CAD build for the part. Positions are in the model's coordinates, mm. A direction names the side the tool comes from. Round coordinates to 2 decimals unless told otherwise and drop trailing zeros. Loops run counter-clockwise (first coordinate to the right, second up) from the corner with the lowest first, then second, coordinate; pieces in that order, holes last. Notation, with made-up numbers: M -29,31 L 22,31 A13 ccw 22,41 Z; hole C 13,37.25 d8. An arc over 180 degrees is marked long. One line per item, written item: value. Start each with the question number.
from build123d import *

# Parameters (mm, degrees)
SCHIZZO1_R                   = 12.1
ESTRUSIONE_ESTRUSIONE1_DEPTH = 1
ESTRUSIONE_ESTRUSIONE2_START = -1.8
SCHIZZO2_R                   = 12.1
SCHIZZO2_R_2                 = 9
ESTRUSIONE_ESTRUSIONE2_DEPTH = 1.8
SCHIZZO3_R                   = 1.925
ESTRUSIONE_ESTRUSIONE3_DEPTH = 11
SCHIZZO4_R                   = 1.7
TAGLIO_ESTRUSIONE1_DEPTH     = 2
TAGLIO_ESTRUSIONE2_START     = -7.2
SCHIZZO5_R                   = 1.925
TAGLIO_ESTRUSIONE2_DEPTH     = 7.2
SCHIZZO6_R                   = 1.425
ESTRUSIONE_ESTRUSIONE4_DEPTH = 3.4
SCHIZZO7_R                   = 1.925
ESTRUSIONE_ESTRUSIONE5_DEPTH = 3.8


with BuildPart() as part:
    # Schizzo1 → Estrusione-Estrusione1 (new body)
    with BuildSketch(Plane.XY):
        with BuildLine():
            Line((-6.171311325, 16.1), (6.171311325, 16.1))
            ThreePointArc((6.171311325, 16.1), (13.651991863, 12.73622021), (16.1, 4.907883736))
            Line((16.1, 4.907883736), (16.1, -13.463208293))
            ThreePointArc((16.1, -13.463208293), (14.572915114, -17.149917336), (10.886206072, -18.677002221))
            Line((10.886206072, -18.677002221), (-10.957517396, -18.677002221))
            ThreePointArc((-10.957517396, -18.677002221), (-14.644226439, -17.149917336), (-16.171311325, -13.463208293))
            Line((-16.171311325, -13.463208293), (-16.171311325, 6.1))
            ThreePointArc((-16.171311325, 6.1), (-13.242379137, 13.171067812), (-6.171311325, 16.1))
        make_face()
        Circle(SCHIZZO1_R, mode=Mode.SUBTRACT)
    extrude(amount=ESTRUSIONE_ESTRUSIONE1_DEPTH)

    # Schizzo2 → Estrusione-Estrusione2 (add)
    with BuildSketch(Plane.XY.offset(1).offset(ESTRUSIONE_ESTRUSIONE2_START)):
        Circle(SCHIZZO2_R)
        Circle(SCHIZZO2_R_2, mode=Mode.SUBTRACT)
    extrude(amount=ESTRUSIONE_ESTRUSIONE2_DEPTH)

    # Schizzo3 → Estrusione-Estrusione3 (add)
    with BuildSketch(Plane(origin=(0, 0, 0), x_dir=(-1, 0, 0), z_dir=(0, 0, -1))):
        with Locations(Location((-10.944459062, 10.817992606, 0), (0, 0, 180))):
            Circle(SCHIZZO3_R)
        with Locations(Location((10.910719744, 10.851964601, 0), (0, 0, 180))):
            Circle(SCHIZZO3_R)
        with Locations(Location((0, -15.38859776, 0), (0, 0, 180))):
            Circle(SCHIZZO3_R)
    extrude(amount=ESTRUSIONE_ESTRUSIONE3_DEPTH)

    # Schizzo4 → Taglio-Estrusione1 (cut)
    with BuildSketch(Plane(origin=(0, 12.776964601, 0), x_dir=(1, 0, 0), z_dir=(0, 1, 0))):
        with BuildLine():
            ThreePointArc((-9.045346347, 5.425199137), (-9.603228747, 6.684392286), (-10.910719744, 7.117136381))
            Line((-10.910719744, 7.117136381), (-10.910719744, 3.733261892))
            ThreePointArc((-10.910719744, 3.733261892), (-9.603228747, 4.166005987), (-9.045346347, 5.425199137))
        make_face()
        with BuildLine():
            Line((-10.910719744, 3.733261892), (-10.910719744, 7.117136381))
            ThreePointArc((-10.910719744, 7.117136381), (-12.445346347, 5.425199137), (-10.910719744, 3.733261892))
        make_face()
        with Locations(Location((10.944459062, 5.5, 0), (0, 0, 270))):
            Circle(SCHIZZO4_R)
    extrude(amount=-TAGLIO_ESTRUSIONE1_DEPTH, mode=Mode.SUBTRACT)

    # Schizzo5 → Taglio-Estrusione2 (cut)
    with BuildSketch(Plane(origin=(0, 0, -11), x_dir=(-1, 0, 0), z_dir=(0, 0, -1)).offset(TAGLIO_ESTRUSIONE2_START)):
        with Locations(Location((0, -15.38859776, 0), (0, 0, 180))):
            Circle(SCHIZZO5_R)
    extrude(amount=TAGLIO_ESTRUSIONE2_DEPTH, mode=Mode.SUBTRACT)

    # Schizzo6 → Estrusione-Estrusione4 (add)
    with BuildSketch(Plane(origin=(0, 0, -3.8), x_dir=(-1, 0, 0), z_dir=(0, 0, -1))):
        with Locations((0, -15.38859776)):
            Circle(SCHIZZO6_R)
    extrude(amount=ESTRUSIONE_ESTRUSIONE4_DEPTH)

    # Schizzo7 → Estrusione-Estrusione5 (add)
    with BuildSketch(Plane(origin=(0, 0, -7.2), x_dir=(-1, 0, 0), z_dir=(0, 0, -1))):
        with Locations(Location((0, -15.38859776, 0), (0, 0, 180))):
            Circle(SCHIZZO7_R)
    extrude(amount=ESTRUSIONE_ESTRUSIONE5_DEPTH)


solid = part.part
(1) Flat gauge pins, fed straight in: P1, Ø6, axis at x = 6.5, y = -1.5, coming from the -Z side; P2, Ø2, axis at x = 10.94, z = -5.5, coming from the +Y side; P3, Ø3, axis at y = -5.5, z = -2, coming from the +X side; P4, Ø6, axis at y = -7, z = -6.5, coming from the -X side. Where does each tip first touch, or does it go through?
(2) Which spindle directions (+Z, -Z, +X, -X, +Y, -Y) get a long thin tool onto all of the face, cutting with end or side? Do faces 1 (the flat face through (0, -17, -3.8)), 2 (the flat face through (0.1, -18.677, 0.5)), 3 (the cylindrical face through (-11.161, 8.943, -5.423)). Say none if no direction does.
(3) Slice it at B-B, the plane y = 0. List the corners of the cut face in (x, z), and give its area (3 significant figures).
(4) Slice it at A-A, the plane x = 0. List the corners of the cut face in (y, z), and give its area (3 significant figures).
(5) Mould opens along X. For faces 4 (the flat face through (16.1, -4.1, 0.5)), 5 (the cylindrical face through (10.69, 8.91, -5.42)), 6 (the flat face through (0, -17, -7.2)), 7 (the cylindrical face through (-1.172, 8.923, 0.087)) say: pulls with the +X half, pulls with the -X half, needs draft (parallel to the pull), parting line crosses it, or undercut.
(6) Probe L1, parallel to Y at x = 0, z = -0.05; L2, parallel to Z at x = -8.5, y = -7; L3, parallel to Y at x = 0, z = 0.1. List the from-to ranges inside material, lowest first.
(7) Slice it at C-C, the plane z = -4.5. List the corners of the cut face in (x, y) (3 decimals), and give its area (3 significant figures).
(8) Slice it at D-D, the plane x = -7.5. List the corners of the cut face in (y, z), and give its area (3 significant figures).
Check result:
1. P1: stops at z = -0.8
1. P2: stops at y = 10.78
1. P3: stops at x = 11.19
1. P4: passes through
2. face 1: none
2. face 2: +Z, -Z, +X, -X, -Y
2. face 3: -Z
3. outline: M -16.17,0 L -12.1,0 L -12.1,-0.8 L -9,-0.8 L -9,1 L -16.17,1 Z; M 9,-0.8 L 12.1,-0.8 L 12.1,0 L 16.1,0 L 16.1,1 L 9,1 Z
3. area: 19.2 mm^2
4. outline: M -18.68,0 L -17.31,0 L -17.31,-3.8 L -16.81,-3.8 L -16.81,-7.2 L -17.31,-7.2 L -17.31,-11 L -13.46,-11 L -13.46,-7.2 L -13.96,-7.2 L -13.96,-3.8 L -13.46,-3.8 L -13.46,0 L -12.1,0 L -12.1,-0.8 L -9,-0.8 L -9,1 L -18.68,1 Z; M 9,-0.8 L 12.1,-0.8 L 12.1,0 L 16.1,0 L 16.1,1 L 9,1 Z
4. area: 60.7 mm^2
5. face 4: pulls with the +X half
5. face 5: undercut
5. face 6: needs draft
5. face 7: undercut
6. L1: y = -17.31 to -13.46, -12.1 to -9, 9 to 12.1
6. L2: z = -0.8 to 1
6. L3: y = -18.68 to -9, 9 to 16.1
7. outline: M -12.172,10.777 L -12.172,12.307 A1.925 ccw long -9.319,11.935 L -9.319,10.777 Z; C 0,-15.389 d2.85; M 9.57,10.777 L 9.57,12.165 A1.925 ccw long 12.319,12.165 L 12.319,10.777 Z
7. area: 19.6 mm^2
8. outline: M -18.68,0 L -9.5,0 L -9.5,-0.8 L -4.97,-0.8 L -4.97,1 L -18.68,1 Z; M 4.97,-0.8 L 9.5,-0.8 L 9.5,0 L 16.01,0 L 16.01,1 L 4.97,1 Z
8. area: 32.0 mm^2
